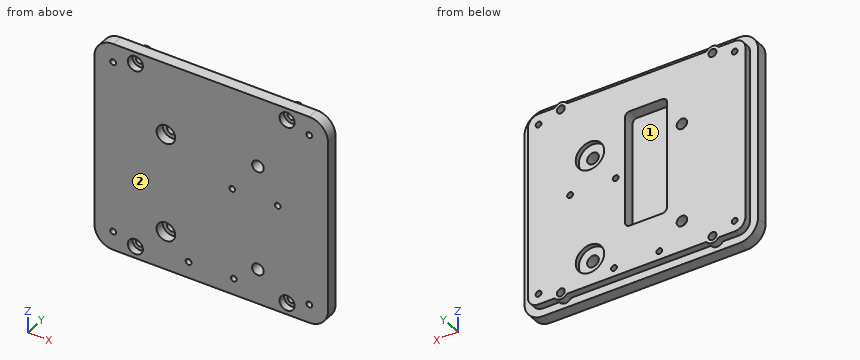
from build123d import *

# Parameters (mm, degrees)
SKETCH1_W                      = 100
SKETCH1_H                      = 90
BOSS_EXTRUDE1_DEPTH            = 8
FILLET1_R                      = 8
SKETCH6_R                      = 6.1
CUT_EXTRUDE1_DEPTH             = 2
SKETCH7_OUTSIDE_W              = 128.954
SKETCH7_OUTSIDE_H              = 118.954
CUT_EXTRUDE2_DEPTH             = 3
M3X0_5_TAPPED_HOLE1_D          = 2.5
M6X1_0_TAPPED_HOLE2_D          = 5
SKETCH12_R                     = 3
SKETCH12_R_2                   = 1.660846167
BOSS_EXTRUDE2_DEPTH            = 3
CBORE_FOR_M3_SHCS1_D           = 3.4
CBORE_FOR_M3_SHCS1_CBORE_D     = 6.5
CBORE_FOR_M3_SHCS1_CBORE_DEPTH = 3
FILLET2_R                      = 1
SKETCH15_W                     = 18
SKETCH15_H                     = 50
CUT_EXTRUDE3_DEPTH             = 5
FILLET3_R                      = 2
CBORE_FOR_M4_SHCS1_D           = 4.5
CBORE_FOR_M4_SHCS1_CBORE_D     = 8
CBORE_FOR_M4_SHCS1_CBORE_DEPTH = 4


with BuildPart() as part:
    # Sketch1 → Boss-Extrude1 (new body)
    with BuildSketch(Plane(origin=(0, 0, 0), x_dir=(1, 0, 0), z_dir=(0, 1, 0))):
        Rectangle(SKETCH1_W, SKETCH1_H)
    extrude(amount=BOSS_EXTRUDE1_DEPTH)

    # Fillet1
    fillet1_edges = [part.edges().sort_by_distance(p)[0] for p in [
        (50, 4, 45),
        (-50, 4, 45),
        (-50, 4, -45),
        (50, 4, -45),
    ]]
    fillet(fillet1_edges, radius=FILLET1_R)

    # Sketch6 → Cut-Extrude1 (cut)
    with BuildSketch(Plane(origin=(0, 8, 0), x_dir=(1, 0, 0), z_dir=(0, 1, 0))):
        with Locations((20, 30)):
            Circle(SKETCH6_R)
        with Locations((20, -15)):
            Circle(SKETCH6_R)
    extrude(amount=-CUT_EXTRUDE1_DEPTH, mode=Mode.SUBTRACT)

    # Sketch7 outside → Cut-Extrude2 (cut)
    with BuildSketch(Plane(origin=(0, 8, 0), x_dir=(1, 0, 0), z_dir=(0, 1, 0))):
        Rectangle(SKETCH7_OUTSIDE_W, SKETCH7_OUTSIDE_H)
        with BuildLine():
            Line((-42, -41.6), (42, -41.6))
            ThreePointArc((42, -41.6), (45.252691193, -40.252691193), (46.6, -37))
            Line((46.6, -37), (46.6, 37))
            ThreePointArc((46.6, 37), (45.252691193, 40.252691193), (42, 41.6))
            Line((42, 41.6), (-42, 41.6))
            ThreePointArc((-42, 41.6), (-45.252691193, 40.252691193), (-46.6, 37))
            Line((-46.6, 37), (-46.6, -37))
            ThreePointArc((-46.6, -37), (-45.252691193, -40.252691193), (-42, -41.6))
        make_face(mode=Mode.SUBTRACT)
    extrude(amount=-CUT_EXTRUDE2_DEPTH, mode=Mode.SUBTRACT)

    # M3x0.5 Tapped Hole1 (through all)
    with Locations(Plane(origin=(0, 8, 0), x_dir=(1, 0, 0), z_dir=(0, 1, 0))):
        with Locations((-42, -37), (-42, 37), (42, 37), (42, -37), (-9.7, 38), (9.7, 38), (28.5, -1), (9, -1)):
            Hole(M3X0_5_TAPPED_HOLE1_D / 2)

    # M6x1.0 Tapped Hole2 (through all)
    with Locations(Plane(origin=(0, 8, 0), x_dir=(1, 0, 0), z_dir=(0, 1, 0))):
        with Locations((20, 30), (20, -15)):
            Hole(M6X1_0_TAPPED_HOLE2_D / 2)

    # Sketch12 → Boss-Extrude2 (add)
    with BuildSketch(Plane(origin=(0, 8, 0), x_dir=(1, 0, 0), z_dir=(0, 1, 0))):
        with Locations((-32.5, 40)):
            Circle(SKETCH12_R)
        with Locations((-32.5, 40)):
            Circle(SKETCH12_R_2, mode=Mode.SUBTRACT)
        with Locations((32.5, 40)):
            Circle(SKETCH12_R)
        with Locations((32.5, 40)):
            Circle(SKETCH12_R_2, mode=Mode.SUBTRACT)
        with Locations((-32.5, -40)):
            Circle(SKETCH12_R)
        with Locations((-32.5, -40)):
            Circle(SKETCH12_R_2, mode=Mode.SUBTRACT)
        with Locations((32.5, -40)):
            Circle(SKETCH12_R)
        with Locations((32.5, -40)):
            Circle(SKETCH12_R_2, mode=Mode.SUBTRACT)
    extrude(amount=-BOSS_EXTRUDE2_DEPTH)

    # CBORE for M3 SHCS1 (through all)
    with Locations(Plane(origin=(0, 0, 0), x_dir=(-1, 0, 0), z_dir=(0, -1, 0))):
        with Locations((32.5, -40), (-32.5, -40), (32.5, 40), (-32.5, 40)):
            CounterBoreHole(CBORE_FOR_M3_SHCS1_D / 2, CBORE_FOR_M3_SHCS1_CBORE_D / 2, CBORE_FOR_M3_SHCS1_CBORE_DEPTH)

    # Fillet2
    fillet2_edges = [part.edges().sort_by_distance(p)[0] for p in [
        (-29.962284492, 6.5, -41.6),
        (-35.037715508, 6.5, -41.6),
        (35.037715508, 6.5, -41.6),
        (29.962284492, 6.5, -41.6),
        (-35.037715508, 6.5, 41.6),
        (-29.962284492, 6.5, 41.6),
        (35.037715508, 6.5, 41.6),
        (29.962284492, 6.5, 41.6),
    ]]
    fillet(fillet2_edges, radius=FILLET2_R)

    # Sketch15 → Cut-Extrude3 (cut)
    with BuildSketch(Plane(origin=(0, 8, 0), x_dir=(1, 0, 0), z_dir=(0, 1, 0))):
        with Locations((-4, -3)):
            Rectangle(SKETCH15_W, SKETCH15_H)
    extrude(amount=-CUT_EXTRUDE3_DEPTH, mode=Mode.SUBTRACT)

    # Fillet3
    fillet3_edges = [part.edges().sort_by_distance(p)[0] for p in [
        (-13, 5.5, 28),
        (-13, 5.5, -22),
        (5, 5.5, -22),
        (5, 5.5, 28),
    ]]
    fillet(fillet3_edges, radius=FILLET3_R)

    # CBORE for M4 SHCS1 (through all)
    with Locations(Plane(origin=(0, 0, 0), x_dir=(-1, 0, 0), z_dir=(0, -1, 0))):
        with Locations((19.4, -14), (19.4, 28.5)):
            CounterBoreHole(CBORE_FOR_M4_SHCS1_D / 2, CBORE_FOR_M4_SHCS1_CBORE_D / 2, CBORE_FOR_M4_SHCS1_CBORE_DEPTH)


solid = part.part
Read the model definition and answer for the solid it produces. Units are mm, in the model's axes. Face numbers are marked on the shaded views. Give positions to 0.01 mm unless a question says otherwise; leave off trailing zeros. Write each loop counter-clockwise with the first axis right and the second up, starting at its lowest first coordinate (ties: lowest second). Pieces come first, ordered by that corner, then holes. Notation, with made-up numbers: (-36, 34) - (-5, 34) arc R31 ccw to (-5, 63) - close; hole circle Ø6 at (-17, 82). An arc over 180 degrees is marked (long way). Answer in a Markdown table with one row per item. Add a question column.
Item 1: Section B-B, the plane z = 40 is taken. Write down the section's boundary in (x, y).
Item 2: Flat-ended cylindrical pins translate along their axes: P1, Ø3.5, axis at x = -39.5, y = 7, coming from the -Z side; P2, Ø5, axis at x = -32.5, z = -40, coming from the -Y side; P3, Ø2.5, axis at y = 6.5, z = -1.5, coming from the +X side. Find the tip coordinate at first contact, or state that the pin passes through.
Item 3: Section C-C, the plane x = 24 is taken. Write down the section's boundary in (y, z).
Item 4: Section A-A, the plane z = -3 is taken. Write down the section's boundary in (x, y).
Item 5: Find the intervals of material crossed by L1, parallel to Z at x = -9.5, y = 5.5; L2, parallel to Z at x = -32.5, y = 5.9; L3, parallel to X at y = 4.25, z = 37, in increasing order.
Item 6: Determine the mould class of the marked faces 1 and 2 for opening direction X: pulls with the +X half, pulls with the -X half, needs draft (parallel to the pull), parting line crosses it, or undercut.
Recorded:
| question | item | result |
|---|---|---|
| 1 | outline | (-49.42, 0) - (-35.75, 0) - (-35.75, 3) - (-34.2, 3) - (-34.2, 8) - (-45.49, 8) - (-45.49, 5) - (-49.42, 5) - close; (-30.8, 3) - (-29.25, 3) - (-29.25, 0) - (29.25, 0) - (29.25, 3) - (30.8, 3) - (30.8, 8) - (-30.8, 8) - close; (34.2, 3) - (35.75, 3) - (35.75, 0) - (49.42, 0) - (49.42, 5) - (45.49, 5) - (45.49, 8) - (34.2, 8) - close |
| 2 | P1 | stops at z = -41.6 |
| 2 | P2 | stops at y = 3 |
| 2 | P3 | stops at x = 46.6 |
| 3 | outline | (0, -45) - (5, -45) - (5, -41.6) - (8, -41.6) - (8, -34.61) - (6, -34.61) - (6, -25.39) - (8, -25.39) - (8, 10.39) - (6, 10.39) - (6, 19.61) - (8, 19.61) - (8, 41.6) - (5, 41.6) - (5, 45) - (0, 45) - close |
| 4 | outline | (-50, 0) - (50, 0) - (50, 5) - (46.6, 5) - (46.6, 8) - (5, 8) - (5, 3) - (-13, 3) - (-13, 8) - (-46.6, 8) - (-46.6, 5) - (-50, 5) - close |
| 5 | L1 | z = -41.6 to -39.23, -36.77 to -22, 28 to 41.6 |
| 5 | L2 | z = -43 to -41.7, -38.3 to 38.3, 41.7 to 43 |
| 5 | L3 | x = -50 to -43.25, -40.75 to 40.75, 43.25 to 50 |
| 6 | face 1 | undercut |
| 6 | face 2 | needs draft |
